```python
from build123d import *

# Parameters (mm, degrees)
BOSS_EXTRUDE1_DEPTH = 125
SKETCH4_W           = 250
SKETCH4_H           = 210
CUT_EXTRUDE2_DEPTH  = 250
BOSS_EXTRUDE2_DEPTH = 15
LPATTERN1_COUNT     = 2
LPATTERN1_PITCH     = 60
LPATTERN1_COL_COUNT = 2
LPATTERN1_COL_PITCH = 60
SKETCH5_W           = 210
SKETCH5_H           = 10
CUT_EXTRUDE3_DEPTH  = 65
SKETCH6_W           = 210
SKETCH6_H           = 10
CUT_EXTRUDE4_DEPTH  = 65


with BuildPart() as part:
    # Sketch1 → Boss-Extrude1 (new, symmetric)
    with BuildSketch(Plane.XY):
        with BuildLine():
            Line((20, 0), (125, 0))
            Line((125, 0), (175, 0))
            Line((175, 0), (175, 170))
            Line((175, 170), (-175, 170))
            Line((-175, 170), (-175, 0))
            Line((-175, 0), (-125, 0))
            Line((-125, 0), (-20, 0))
            ThreePointArc((-20, 0), (0, 20), (20, 0))
        make_face()
    extrude(amount=BOSS_EXTRUDE1_DEPTH, both=True)

    # Sketch4 → Cut-Extrude2 (cut)
    with BuildSketch(Plane(origin=(0, 170, 0), x_dir=(1, 0, 0), z_dir=(0, 1, 0))):
        Rectangle(SKETCH4_W, SKETCH4_H)
    extrude(amount=-CUT_EXTRUDE2_DEPTH, mode=Mode.SUBTRACT)

    # Sketch3 → Boss-Extrude2 (add, symmetric)
    with BuildSketch(Plane.XY):
        with BuildLine():
            Line((125, 0), (125, 30))
            Line((125, 30), (90.138781887, 30))
            ThreePointArc((90.138781887, 30), (0, 95), (-90.138781887, 30))
            Line((-90.138781887, 30), (-125, 30))
            Line((-125, 30), (-125, 0))
            Line((-125, 0), (-20, 0))
            ThreePointArc((-20, 0), (0, 20), (20, 0))
            Line((20, 0), (125, 0))
        make_face()
    boss_extrude2 = extrude(amount=BOSS_EXTRUDE2_DEPTH, both=True)

    # LPattern1: Boss-Extrude2 ×2
    with Locations(*[(0, 0, i * LPATTERN1_PITCH) for i in range(1, LPATTERN1_COUNT)]):
        add(boss_extrude2)

    # LPattern1 col: Boss-Extrude2 ×2
    with Locations(*[(0, 0, -i * LPATTERN1_COL_PITCH) for i in range(1, LPATTERN1_COL_COUNT)]):
        add(boss_extrude2)

    # Sketch5 → Cut-Extrude3 (cut)
    with BuildSketch(Plane(origin=(175, 0, 0), x_dir=(0, 0, -1), z_dir=(1, 0, 0))):
        with Locations((0, 5)):
            Rectangle(SKETCH5_W, SKETCH5_H)
    extrude(amount=-CUT_EXTRUDE3_DEPTH, mode=Mode.SUBTRACT)

    # Sketch6 → Cut-Extrude4 (cut)
    with BuildSketch(Plane.ZY.offset(175)):
        with Locations((0, 5)):
            Rectangle(SKETCH6_W, SKETCH6_H)
    extrude(amount=-CUT_EXTRUDE4_DEPTH, mode=Mode.SUBTRACT)


solid = part.part
```
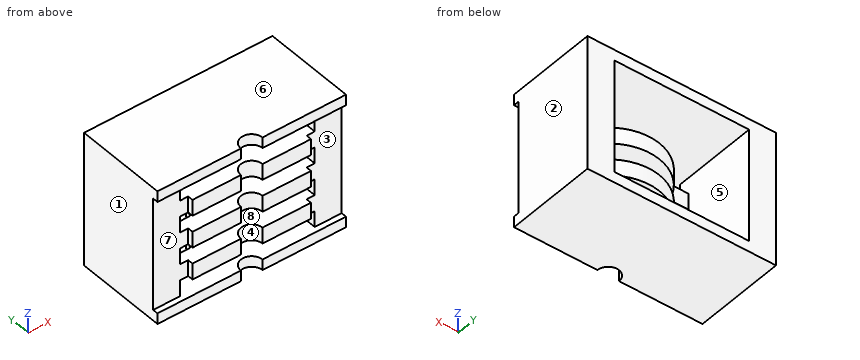
The listing builds one solid part. Answer for the finished solid, in the listing's coordinates (mm). Face numbers are marked on the shaded views. A direction names the side the tool comes from. Round coordinates to 2 decimals unless told otherwise and drop trailing zeros. Loops run counter-clockwise (first coordinate to the right, second up) from the corner with the lowest first, then second, coordinate; pieces in that order, holes last. Notation, with made-up numbers: (61, 2) - (91, 2) arc R26 ccw to (91, 29) - close; hole circle Ø2 at (35, 37.5). An arc over 180 degrees is marked (long way). Return JSON: item names as keys, results as strings. Group by question number.
1. The part is cut by section A-A on x = -96.5. Determine the outline of the cut face in (y, z).
2. Each of these flat-tipped pins is pushed along its axis until it touches: P1, Ø3, axis at y = 6.5, z = -64.5, coming from the +X side; P2, Ø15, axis at x = 108.5, z = -62, coming from the +Y side; P3, Ø11, axis at y = 3.5, z = -56.5, coming from the -X side. Where does it stop, or does it pass through?
3. Which of the six approach directions +Z, -Z, +X, -X, +Y, -Y give full straight-line access (tool end or side, diameter ignored) to the marked faces 5, 6, 7 and 8?
4. The part is cut by section B-B on z = 19.5. Determine the outline of the cut face in (x, y).
5. The mould has two halves that part along X. Classify the marked faces 1, 2, 3 and 4: pulls with the +X half, pulls with the -X half, needs draft (parallel to the pull), parting line crosses it, or undercut.
6. Consider probe 1 along Z at (x, y) = (-38.5, 147); probe 2 along X at (y, z) = (89.5, -30); probe 3 along Y at (x, z) = (108, 63). Determine where each line is inside the solid, lowest interval first.
7. The part is cut by section C-C on y = 78. Determine the outline of the cut face in (x, z).
8. The part is cut by section D-D on y = 120.5. Determine the outline of the cut face in (x, z).
Resolved:
{
 "1": {"outline": "(0, -125) - (170, -125) - (170, -105) - (0, -105) - close; (0, -75) - (30, -75) - (30, -45) - (0, -45) - close; (0, -15) - (30, -15) - (30, 15) - (0, 15) - close; (0, 45) - (30, 45) - (30, 75) - (0, 75) - close; (0, 105) - (170, 105) - (170, 125) - (0, 125) - close"},
 "2": {"P1": "stops at x = 110", "P2": "stops at y = 30", "P3": "stops at x = -110"},
 "3": {"face 5": "+Y", "face 6": "+Z, +X, -X, +Y, -Y", "face 7": "-X, -Y", "face 8": "+Y, -Y"},
 "4": {"outline": "(-175, 10) - (-125, 10) - (-125, 170) - (-175, 170) - close; (125, 10) - (175, 10) - (175, 170) - (125, 170) - close"},
 "5": {"face 1": "pulls with the -X half", "face 2": "pulls with the +X half", "face 3": "needs draft", "face 4": "undercut"},
 "6": {"probe 1": "z = -125 to -105, 105 to 125", "probe 2": "x = -175 to -125, 125 to 175", "probe 3": "y = 0 to 30"},
 "7": {"outline": "(-175, -125) - (175, -125) - (175, 125) - (-175, 125) - close; (-54.23, -75) - (54.23, -75) - (54.23, -45) - (-54.23, -45) - close; (-54.23, -15) - (54.23, -15) - (54.23, 15) - (-54.23, 15) - close; (-54.23, 45) - (54.23, 45) - (54.23, 75) - (-54.23, 75) - close; hole (-125, -105) - (125, -105) - (125, 105) - (-125, 105) - close"},
 "8": {"outline": "(-175, -125) - (175, -125) - (175, 125) - (-175, 125) - close; hole (-125, -105) - (125, -105) - (125, 105) - (-125, 105) - close"}
}
